```python
from build123d import *

# Parameters (mm, degrees)
SKETCH1_W           = 20
SKETCH1_H           = 40
BOSS_EXTRUDE1_DEPTH = 5
SKETCH2_W           = 20
SKETCH2_H           = 9.75
BOSS_EXTRUDE2_DEPTH = 10
SKETCH3_R           = 1.75
CUT_EXTRUDE1_DEPTH  = 5
SKETCH4_R           = 3.363406012
CUT_EXTRUDE2_DEPTH  = 3
SKETCH5_R           = 1.75
CUT_EXTRUDE3_DEPTH  = 8
SKETCH6_W           = 6
SKETCH6_H           = 10
CUT_EXTRUDE4_DEPTH  = 3
SKETCH7_R           = 1.75
CUT_EXTRUDE5_DEPTH  = 3
FILLET1_R           = 5


with BuildPart() as part:
    # Sketch1 → Boss-Extrude1 (new body)
    with BuildSketch(Plane(origin=(0, 0, 0), x_dir=(1, 0, 0), z_dir=(0, 1, 0))):
        Rectangle(SKETCH1_W, SKETCH1_H)
    extrude(amount=BOSS_EXTRUDE1_DEPTH)

    # Sketch2 → Boss-Extrude2 (add)
    with BuildSketch(Plane.XZ):
        with Locations((0, 15.125)):
            Rectangle(SKETCH2_W, SKETCH2_H)
        with Locations((0, -15.125)):
            Rectangle(SKETCH2_W, SKETCH2_H)
    extrude(amount=BOSS_EXTRUDE2_DEPTH)

    # Sketch3 → Cut-Extrude1 (cut)
    with BuildSketch(Plane(origin=(0, 5, 0), x_dir=(1, 0, 0), z_dir=(0, 1, 0))):
        with Locations(Location((-7.5, -8, 0), (0, 0, 270))):
            Circle(SKETCH3_R)
        with Locations(Location((-7.5, 8, 0), (0, 0, 270))):
            Circle(SKETCH3_R)
        with Locations(Location((7.5, -8, 0), (0, 0, 270))):
            Circle(SKETCH3_R)
        with Locations(Location((7.5, 8, 0), (0, 0, 270))):
            Circle(SKETCH3_R)
    extrude(amount=-CUT_EXTRUDE1_DEPTH, mode=Mode.SUBTRACT)

    # Sketch4 → Cut-Extrude2 (cut)
    with BuildSketch(Plane.XZ):
        with Locations((7.5, 8)):
            Circle(SKETCH4_R)
        with Locations((-7.5, 8)):
            Circle(SKETCH4_R)
        with Locations((-7.5, -8)):
            Circle(SKETCH4_R)
        with Locations((7.5, -8)):
            Circle(SKETCH4_R)
    extrude(amount=-CUT_EXTRUDE2_DEPTH, mode=Mode.SUBTRACT)

    # Sketch5 → Cut-Extrude3 (cut)
    with BuildSketch(Plane.XZ.offset(10)):
        with Locations(Location((-5, -15, 0), (0, 0, 270))):
            Circle(SKETCH5_R)
        with Locations(Location((5, -15, 0), (0, 0, 270))):
            Circle(SKETCH5_R)
        with Locations(Location((-5, 15, 0), (0, 0, 270))):
            Circle(SKETCH5_R)
        with Locations(Location((5, 15, 0), (0, 0, 270))):
            Circle(SKETCH5_R)
    extrude(amount=-CUT_EXTRUDE3_DEPTH, mode=Mode.SUBTRACT)

    # Sketch6 → Cut-Extrude4 (cut)
    with BuildSketch(Plane.XZ.offset(2)):
        with Locations((-5, -15)):
            Rectangle(SKETCH6_W, SKETCH6_H)
        with Locations((5, -15)):
            Rectangle(SKETCH6_W, SKETCH6_H)
        with Locations((5, 15)):
            Rectangle(SKETCH6_W, SKETCH6_H)
        with Locations((-5, 15)):
            Rectangle(SKETCH6_W, SKETCH6_H)
    extrude(amount=CUT_EXTRUDE4_DEPTH, mode=Mode.SUBTRACT)

    # Sketch7 → Cut-Extrude5 (cut)
    with BuildSketch(Plane.XZ.offset(2)):
        with Locations(Location((-5, -15, 0), (0, 0, 270))):
            Circle(SKETCH7_R)
        with Locations(Location((5, -15, 0), (0, 0, 270))):
            Circle(SKETCH7_R)
        with Locations(Location((5, 15, 0), (0, 0, 270))):
            Circle(SKETCH7_R)
        with Locations(Location((-5, 15, 0), (0, 0, 270))):
            Circle(SKETCH7_R)
    extrude(amount=-CUT_EXTRUDE5_DEPTH, mode=Mode.SUBTRACT)

    # Fillet1
    # the kernel refuses this fillet: 5 mm, written as the material it takes off along each edge
    with BuildSketch(Plane(origin=(-10, 17.5, -20), x_dir=(0, 0, 1), z_dir=(0, -1, 0)), Plane(origin=(10, -22.5, -20), x_dir=(0, 0, 1), z_dir=(0, 1, 0)), Plane(origin=(-10, 17.5, 20), x_dir=(1, 0, 0), z_dir=(0, -1, 0)), Plane(origin=(10, -22.5, 20), x_dir=(-1, 0, 0), z_dir=(0, 1, 0))) as fillet1_piece_1:
        with BuildLine():
            CenterArc((FILLET1_R, -FILLET1_R), FILLET1_R, 90, 90)
            Line((0, -FILLET1_R), (0, 0))
            Line((0, 0), (FILLET1_R, 0))
        make_face()
    extrude(amount=40, mode=Mode.SUBTRACT)


solid = part.part
```
Build history of the part. All positions in model axes, mm. A direction names the side the tool comes from. Round coordinates to 2 decimals unless told otherwise and drop trailing zeros. Write each loop counter-clockwise with the first axis right and the second up, starting at its lowest first coordinate (ties: lowest second). Pieces come first, ordered by that corner, then holes.
1) Drill centre lines: probe 1 along X at (y, z) = (3.8, -8); probe 2 along Y at (x, z) = (3.75, -18); probe 3 along Z at (x, y) = (-8, -7.5). Where is each one in solid material? Low to high.
2) Band-saw the part on C-C, the plane x = 1. List the corners of the cut face in (y, z).
3) Pin check, flat tips, straight feed: pin 1 (1.5 mm diameter, centred on y = -3, z = -16, fed in from +X); pin 2 (1 mm diameter, centred on x = 6, z = -15.5, fed in from -Y). Stop position of each tip, or through.
4) 3-axis set-ups, long thin cutter, end or side, ignore diameter. For faces 1 (the flat face through (3, -2, -15)), 2 (the cylindrical face through (9, -3, -18)), 3 (the flat face through (0, 0, 0)), 4 (the cylindrical face through (3.45, -7.54, 14.19)), 5 (the flat face through (5.7, 3, 7.3)): which of +Z, -Z, +X, -X, +Y, -Y reach the whole face in a straight line?
5) Band-saw the part on A-A, the plane z = -8. List the corners of the cut face in (x, y).
6) Band-saw the part on B-B, the plane y = -4. List the corners of the cut face in (x, z), and give its area (3 significant figures).
7) Mould opens along X. For faces 6 (the flat face through (-6, 3, -6)), 7 (the flat face through (0, -3, -20)), 8 (the flat face through (-10, 1, 0)), 9 (the flat face through (3.6, -5, 16.3)) say: +X half, -X half, draft (parallel to the pull), parting line (faces both ways), or undercut.
8) Band-saw the part on D-D, the plane x = 7.5. Give the number of separate pieces and of enclosed holes in the cut face, and give its area (3 significant figures).
Ans:
1. probe 1: x = -10 to -9.25, -5.75 to 5.75, 9.25 to 10
1. probe 2: y = -10 to -5, -2 to 5
1. probe 3: z = -19 to -10.25, 10.25 to 19
2. outline: (-10, -20) - (5, -20) - (5, 20) - (-10, 20) - (-10, 10.25) - (0, 10.25) - (0, -10.25) - (-10, -10.25) - close
3. pin 1: stops at x = 9.99
3. pin 2: stops at y = 1
4. face 1: +Z, -Z
4. face 2: -Z, +X, +Y, -Y
4. face 3: +X, -X, -Y
4. face 4: -Y
4. face 5: none
5. outline: (-10, 3) - (-9.25, 3) - (-9.25, 5) - (-10, 5) - close; (-5.75, 3) - (-4.14, 3) - (-4.14, 0) - (4.14, 0) - (4.14, 3) - (5.75, 3) - (5.75, 5) - (-5.75, 5) - close; (9.25, 3) - (10, 3) - (10, 5) - (9.25, 5) - close
6. outline: (-10, -15) arc R5 ccw to (-8, -19) - (-8, -10.25) - (-10, -10.25) - close; (-10, 10.25) - (-8, 10.25) - (-8, 19) arc R5 ccw to (-10, 15) - close; (-2, -20) - (2, -20) - (2, -10.25) - (-2, -10.25) - close; (-2, 10.25) - (2, 10.25) - (2, 20) - (-2, 20) - close; (8, -19) arc R5 ccw to (10, -15) - (10, -10.25) - (8, -10.25) - close; (8, 10.25) - (10, 10.25) - (10, 15) arc R5 ccw to (8, 19) - close
6. area: 138 mm2
7. face 6: undercut
7. face 7: draft
7. face 8: -X half
7. face 9: undercut
8. separate pieces: 5
8. enclosed holes: 0
8. area: 266 mm2
